Can you work these out from the model? Positions are in its coordinate system, mm. Face numbers are marked on the shaded views. A direction names the side the tool comes from. Coordinates: 2 decimals unless noted, no trailing zeros. Order: outer loops, then holes, each group sorted by start corner. A loop starts at its lowest first (then second) coordinate and runs counter-clockwise, first axis right, second up. Notation, with made-up numbers: (6.5, -15.5) - (55.5, -15.5) arc R18 ccw to (55.5, 10.5) - close; hole circle Ø11 at (6.25, -38). An arc over 180 degrees is marked (long way). Use a Markdown table: item, result. Add a question column.
(1) I want a section at C-C (y = -67.5). List the corners of the cut face in (x, z) for me, and give its area (3 significant figures).
(2) On a 3-axis mill with a long thin cutter (end or side, diameter ignored), from which of +Z, -Z, +X, -X, +Y, -Y can I reach the whole of each face in a straight line? I mean the marked faces 1 and 2. Say none if no direction works.
(3) I want a section at A-A (z = 60.5). List the corners of the cut face in (x, y) for me (3 decimals), and give its area (3 significant figures).
(4) I want a section at B-B (x = 46.5). List the corners of the cut face in (y, z) for me (3 decimals).
(5) If I drill on L1, parallel to Y at x = 21, z = 7.5 (3 decimals); L2, parallel to X at y = -31, z = 70; L3, parallel to Z at x = 122, y = -19.5, over which ranges is the centre line in solid material (lowest first)? Write a range as [from, to].
(6) We'd pull the mould along X, two halves only. Please class the marked faces 3, 4 and 5: pulls with the +X half, pulls with the -X half, needs draft (parallel to the pull), parting line crosses it, or undercut.
(7) For pin 1 Ø1 at (x, z) = (58, 21.5) entering from +Y; pin 2 Ø1.5 at (x, y) = (78.5, -26) entering from -Z; pin 3 Ø1.6 at (x, y) = (69, 1.5) entering from -Z, each with a flat end and sliding along its axis, tell me the tip position at first contact or that it passes through.
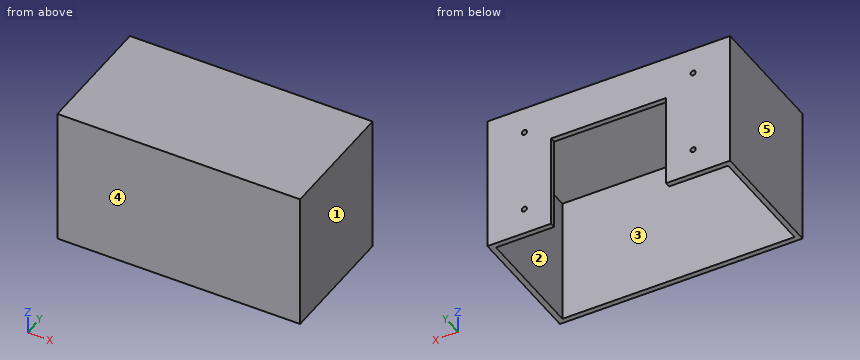
```python
from build123d import *

# Parameters (mm, degrees)
SKETCH1_W           = 146.05
SKETCH1_H           = 76.2
SKETCH1_W_2         = 139.7
SKETCH1_H_2         = 69.85
BOSS_EXTRUDE1_DEPTH = 76.2
SKETCH2_W           = 146.05
SKETCH2_H           = 76.2
BOSS_EXTRUDE2_DEPTH = 6.35
SKETCH3_R           = 1.55
CUT_EXTRUDE1_DEPTH  = 6.35
SKETCH4_W           = 69.251410207
SKETCH4_H           = 56.45274813
CUT_EXTRUDE2_DEPTH  = 25.4


with BuildPart() as part:
    # Sketch1 → Boss-Extrude1 (new body)
    with BuildSketch(Plane.XY):
        with Locations((70.004169971, -34.925)):
            Rectangle(SKETCH1_W, SKETCH1_H)
        with Locations((69.85, -34.925)):
            Rectangle(SKETCH1_W_2, SKETCH1_H_2, mode=Mode.SUBTRACT)
    extrude(amount=BOSS_EXTRUDE1_DEPTH)

    # Sketch2 → Boss-Extrude2 (add)
    with BuildSketch(Plane.XY.offset(76.2)):
        with Locations((70.004169971, -34.925)):
            Rectangle(SKETCH2_W, SKETCH2_H)
    extrude(amount=BOSS_EXTRUDE2_DEPTH)

    # Sketch3 → Cut-Extrude1 (cut)
    with BuildSketch(Plane(origin=(0, 3.175, 0), x_dir=(1, 0, 0), z_dir=(0, 1, 0))):
        with Locations(Location((19.204169971, -15.875, 0), (0, 0, 270))):
            Circle(SKETCH3_R)
        with Locations(Location((120.804169971, -15.875, 0), (0, 0, 270))):
            Circle(SKETCH3_R)
        with Locations(Location((120.804169971, -66.675, 0), (0, 0, 270))):
            Circle(SKETCH3_R)
        with Locations(Location((19.204169971, -66.675, 0), (0, 0, 270))):
            Circle(SKETCH3_R)
    extrude(amount=-CUT_EXTRUDE1_DEPTH, mode=Mode.SUBTRACT)

    # Sketch4 → Cut-Extrude2 (cut)
    with BuildSketch(Plane(origin=(0, 3.175, 0), x_dir=(1, 0, 0), z_dir=(0, 1, 0))):
        with Locations((70.062674023, -28.226374065)):
            Rectangle(SKETCH4_W, SKETCH4_H)
    extrude(amount=-CUT_EXTRUDE2_DEPTH, mode=Mode.SUBTRACT)


solid = part.part
```
Answers follow:
| question | item | result |
|---|---|---|
| 1 | outline | (-3.02, 0) - (0, 0) - (0, 76.2) - (139.7, 76.2) - (139.7, 0) - (143.03, 0) - (143.03, 82.55) - (-3.02, 82.55) - close |
| 1 | area | 1,410 mm² |
| 2 | face 1 | +Z, -Z, +X, +Y, -Y |
| 2 | face 2 | -Z |
| 3 | outline | (-3.021, -73.025) - (143.029, -73.025) - (143.029, 3.175) - (-3.021, 3.175) - close; hole (0, -69.85) - (139.7, -69.85) - (139.7, 0) - (0, 0) - close |
| 3 | area | 1,370 mm² |
| 4 | outline | (-73.025, 0) - (-69.85, 0) - (-69.85, 76.2) - (0, 76.2) - (0, 56.453) - (3.175, 56.453) - (3.175, 82.55) - (-73.025, 82.55) - close |
| 5 | L1 | y = [-73.025, -69.85], [0, 3.175] |
| 5 | L2 | x = [-3.02, 0], [139.7, 143.03] |
| 5 | L3 | z = [76.2, 82.55] |
| 6 | face 3 | undercut |
| 6 | face 4 | needs draft |
| 6 | face 5 | pulls with the -X half |
| 7 | pin 1 | stops at y = -69.85 |
| 7 | pin 2 | stops at z = 76.2 |
| 7 | pin 3 | stops at z = 56.45 |
